from build123d import *

# Parameters (mm, degrees)
F0_R     = 11.1
F1_DEPTH = 7
F2_R     = 5


with BuildPart() as f1:
    # F0 (on Top) → F1 (new body)
    with BuildSketch(Plane.XY):
        with BuildLine():
            Line((19.980762, 25.392305), (0, 60))
            Line((0, 60), (-19.980762, 25.392305))
            ThreePointArc((-19.980762, 25.392305), (-15.588457, 9), (-31.980762, 4.607695))
            Line((-31.980762, 4.607695), (-51.961524, -30))
            Line((-51.961524, -30), (-12, -30))
            ThreePointArc((-12, -30), (0, -18), (12, -30))
            Line((12, -30), (51.961524, -30))
            Line((51.961524, -30), (31.980762, 4.607695))
            ThreePointArc((31.980762, 4.607695), (15.588457, 9), (19.980762, 25.392305))
        make_face()
        with Locations((-25.980762, -15)):
            Circle(F0_R, mode=Mode.SUBTRACT)
        with Locations((25.980762, -15)):
            Circle(F0_R, mode=Mode.SUBTRACT)
        Circle(F0_R, mode=Mode.SUBTRACT)
        with Locations((0, 30)):
            Circle(F0_R, mode=Mode.SUBTRACT)
    extrude(amount=F1_DEPTH)

    # F2
    f2_edges = [f1.edges().sort_by_distance(p)[0] for p in [
        (0, 60, 3.5),
        (51.961524, -30, 3.5),
        (-51.961524, -30, 3.5),
    ]]
    fillet(f2_edges, radius=F2_R)


solid = f1.part
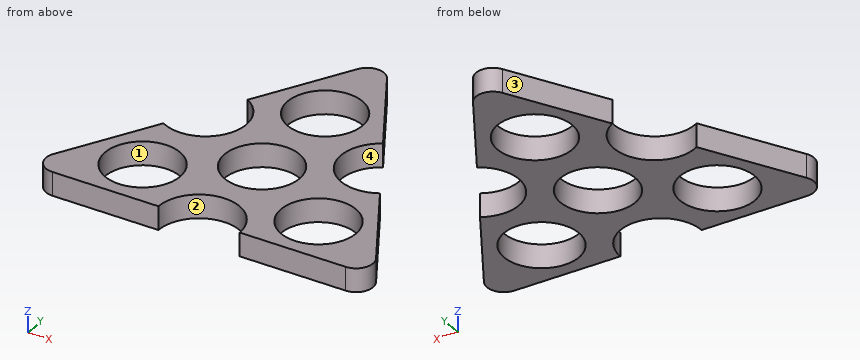
Can you work these out from the model? Positions are in its coordinate system, mm. Face numbers are marked on the shaded views. Coordinates: 2 decimals unless noted, no trailing zeros. Loops run counter-clockwise (first coordinate to the right, second up) from the corner with the lowest first, then second, coordinate; pieces in that order, holes last. Notation, with made-up numbers: (20, 81) - (31, 81) arc R27 cw to (31, 110) - close; hole circle Ø7 at (68.5, 40). An arc over 180 degrees is marked (long way). Put each result on its own line as item: value. Start each with the question number.
Item 1: Suppose I cut it at B-B (y = -24). Please give me the cut outline in (x, z).
Item 2: Suppose I cut it at D-D (y = 30). Please give me the cut outline in (x, z), and give its area (3 significant figures).
Item 3: Suppose I cut it at A-A (x = 0). Please give me the cut outline in (y, z).
Item 4: If I drill on line 1 along Y through (x, z) = (0, 4.5); line 2 along X through (y, z) = (-14, 6.25); line 3 along Y through (x, z) = (5.5, 4.5), over which ranges is the centre line in solid material (lowest first)?
Item 5: Suppose I cut it at C-C (z = 2). Please give me the cut outline in (x, y), and give its area (3 significant figures).
Item 6: For pin 1 (20 mm diameter, centred on x = 0, y = 30, fed in from +Z); pin 2 (2 mm diameter, centred on y = 27.5, z = 2.5, fed in from -X); pin 3 (1.5 mm diameter, centred on y = 22.5, z = 4, fed in from +X); pin 4 (1.5 mm diameter, centred on y = 14.5, z = 2.5, fed in from -X), each with a flat end and sliding along its axis, tell me the tip position at first contact or that it passes through.
Item 7: If we mould it in two halves opening along Y, with no side actions, what happens to the marked faces 1, 2, 3 and 4? For each: +Y half, -Y half, draft (parallel to the pull), parting line (faces both ways), or undercut.
Here are the results:
1. outline: (-48.2, 0) - (-32.48, 0) - (-32.48, 7) - (-48.2, 7) - close; (-19.48, 0) - (-10.39, 0) - (-10.39, 7) - (-19.48, 7) - close; (10.39, 0) - (19.48, 0) - (19.48, 7) - (10.39, 7) - close; (32.48, 0) - (48.2, 0) - (48.2, 7) - (32.48, 7) - close
2. outline: (-17.32, 0) - (-11.1, 0) - (-11.1, 7) - (-17.32, 7) - close; (11.1, 0) - (17.32, 0) - (17.32, 7) - (11.1, 7) - close
2. area: 87.1 mm²
3. outline: (-18, 0) - (-11.1, 0) - (-11.1, 7) - (-18, 7) - close; (11.1, 0) - (18.9, 0) - (18.9, 7) - (11.1, 7) - close; (41.1, 0) - (55, 0) - (55, 7) - (41.1, 7) - close
4. line 1: -18 to -11.1, 11.1 to 18.9, 41.1 to 55
4. line 2: -42.72 to -37.04, -14.93 to 14.93, 37.04 to 42.72
4. line 3: -19.33 to -9.64, 9.64 to 20.36, 39.64 to 50.47
5. outline: (-47.63, -22.5) arc R5 ccw to (-43.3, -30) - (-12, -30) arc R12 cw to (12, -30) - (43.3, -30) arc R5 ccw to (47.63, -22.5) - (31.98, 4.61) arc R12 cw to (19.98, 25.39) - (4.33, 52.5) arc R5 ccw to (-4.33, 52.5) - (-19.98, 25.39) arc R12 cw to (-31.98, 4.61) - close; hole circle Ø22.2 at (-25.98, -15); hole circle Ø22.2 at (0, 0); hole circle Ø22.2 at (0, 30); hole circle Ø22.2 at (25.98, -15)
5. area: 2,400 mm²
6. pin 1: through
6. pin 2: x = -19.34
6. pin 3: x = 17.27
6. pin 4: x = -14.05
7. face 1: undercut
7. face 2: -Y half
7. face 3: +Y half
7. face 4: undercut
